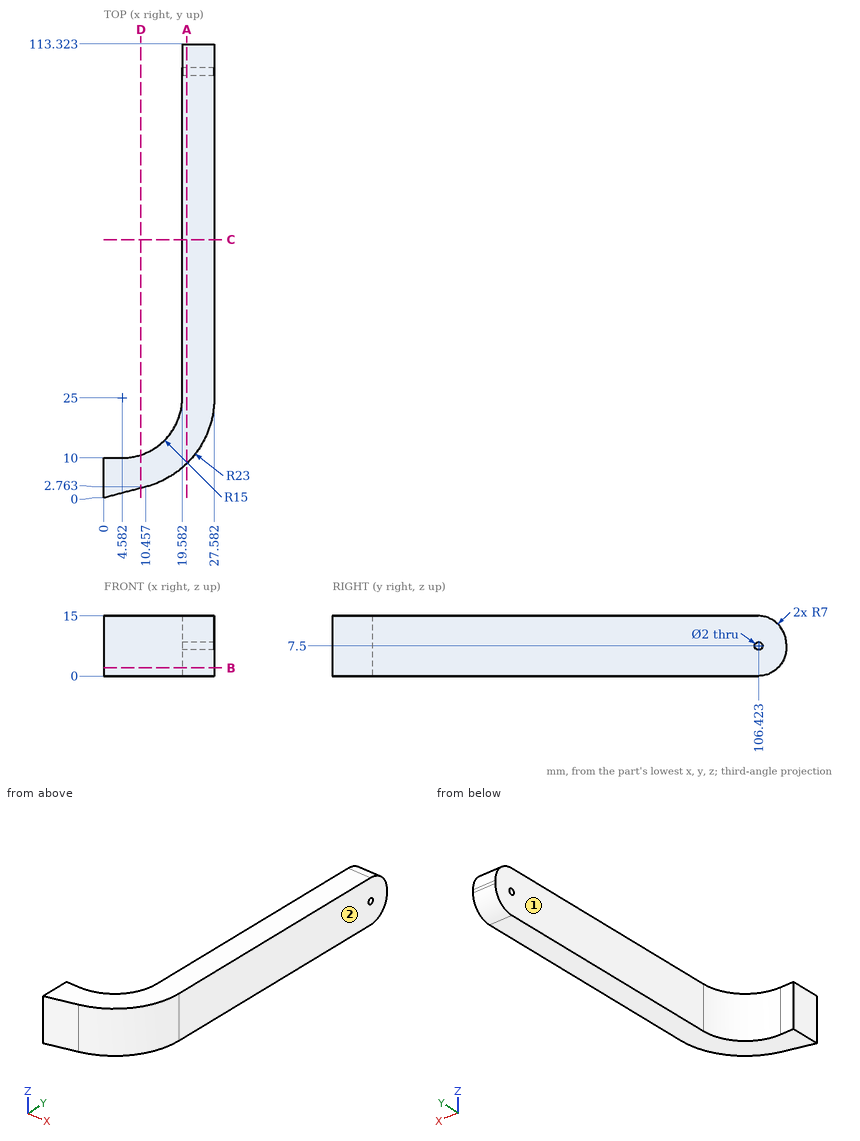
Input: dimensioned drawing with shaded views. Units: mm. Origin: part minimum x, y, z. A direction names the side the tool comes from. Coordinates: 2 decimals unless noted, no trailing zeros. Order: outer loops, then holes, each group sorted by start corner. A loop starts at its lowest first (then second) coordinate and runs counter-clockwise, first axis right, second up.
(1) Access query for the marked faces 1 and 2. Directions: +Z, -Z, +X, -X, +Y, -Y. A direction counts if a zero-diameter tool reaches every point of the face in a straight line with its end or side. Return the directions, or none.
(2) Section query B-B (z = 2). Return the cut outline in (x, y).
(3) Section query C-C (y = 64.5). Return the cut outline in (x, z).
(4) First-contact query: pin 1 (1.6 mm diameter, centred on y = 106.42, z = 7.5, fed in from -X); pin 2 (2.5 mm diameter, centred on x = 2, z = 11, fed in from +Y); pin 3 (5 mm diameter, centred on x = 11.5, z = 4, fed in from +Y) (1 decimal); pin 4 (1 mm diameter, centred on y = 60, z = 9.5, fed in from -X). Flat tips, straight axial feed; report the tip coordinate or a pass-through.
(5) Material intervals for probe 1 along X at (y, z) = (36, 13.5); probe 2 along Y at (x, z) = (22.25, 7.5) (1 decimal); probe 3 along Y at (x, z) = (24, 7.5) (1 decimal), sorted ascending.
(6) Section query D-D (x = 9.25). Return the cut outline in (y, z) (1 decimal).
(7) Section query A-A (x = 20.75). Return the cut outline in (y, z), plus the area to 3 significant figures.
Solution:
1. face 1: +Z, -Z, -X, +Y
1. face 2: +Z, -Z, +X, +Y, -Y
2. outline: (0, 0) - (10.46, 2.76) arc R23 ccw to (27.58, 25) - (27.58, 111.22) - (19.58, 111.22) - (19.58, 25) arc R15 cw to (4.58, 10) - (0, 10) - close
3. outline: (19.58, 0) - (27.58, 0) - (27.58, 15) - (19.58, 15) - close
4. pin 1: passes through
4. pin 2: stops at y = 10
4. pin 3: stops at y = 13.3
4. pin 4: stops at x = 19.58
5. probe 1: x = 19.58 to 27.58
5. probe 2: y = 10.3 to 105.4, 107.4 to 113.3
5. probe 3: y = 12.7 to 105.4, 107.4 to 113.3
6. outline: (2.4, 0) - (10.7, 0) - (10.7, 15) - (2.4, 15) - close
7. outline: (8.64, 0) - (106.32, 0) arc R7 ccw to (113.32, 7) - (113.32, 8) arc R7 ccw to (106.32, 15) - (8.64, 15) - close; hole circle Ø2 at (106.42, 7.5)
7. area: 1,550 mm2
